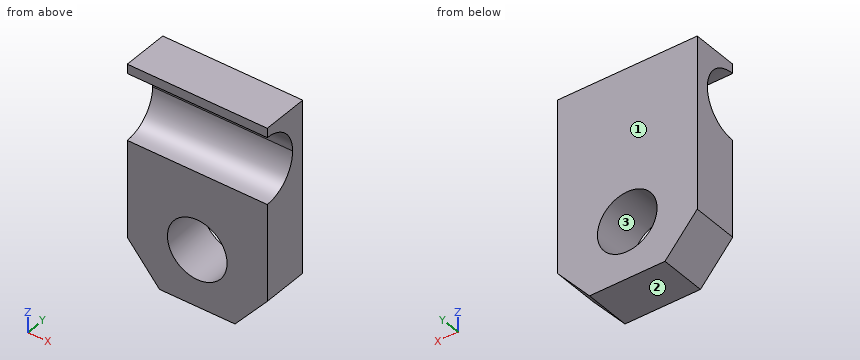
```python
from build123d import *

# Parameters (mm, degrees)
F0_W      = 38.1
F0_H      = 57.15
F1_DEPTH  = 12.7
F3_DEPTH  = 25.4
F7_DEPTH  = 101.6
F9_DEPTH  = 2.54
F10_R     = 8.114992
F11_DEPTH = 25.4


with BuildPart() as f1:
    # F0 (on Front) → F1 (new body)
    with BuildSketch(Plane.XZ):
        Rectangle(F0_W, F0_H)
    extrude(amount=F1_DEPTH)

    # F2 (on face) → F3 (cut)
    with BuildSketch(Plane.XZ.offset(12.7)):
        Polygon((19.05, -18.421547), (10.264741, -28.575), (19.05, -28.575), align=None)
        Polygon((-19.05, -28.575), (-10.264741, -28.575), (-19.05, -18.421547), align=None)
    extrude(amount=-F3_DEPTH, mode=Mode.SUBTRACT)

    # F5 (on face) → F7 (cut)
    with BuildSketch(Plane.YZ.offset(19.05)):
        with BuildLine():
            ThreePointArc((-12.7, 7.877494), (-6.281125, 10.536279), (-3.62234, 16.955154))
            ThreePointArc((-3.62234, 16.955154), (-6.281125, 23.374029), (-12.7, 26.032814))
            Line((-12.7, 26.032814), (-12.7, 7.877494))
        make_face()
        with BuildLine():
            Line((-12.7, 7.877494), (-12.7, 26.032814))
            ThreePointArc((-12.7, 26.032814), (-21.77766, 16.955154), (-12.7, 7.877494))
        make_face()
    extrude(amount=-F7_DEPTH, mode=Mode.SUBTRACT)

    # F8 (on face) → F9 (join)
    with BuildSketch(Plane(origin=(0, 0, 0), x_dir=(-1, 0, 0), z_dir=(0, 1, 0))):
        Polygon((-19.05, 28.575), (-19.05, -18.421547), (-10.264741, -28.575), (10.264741, -28.575), (19.05, -18.421547), (19.05, 28.575), align=None)
    extrude(amount=-F9_DEPTH)

    # F10 (on face) → F11 (cut)
    with BuildSketch(Plane.XZ.offset(12.7)):
        with Locations((0, -13.105877)):
            Circle(F10_R)
    extrude(amount=-F11_DEPTH, mode=Mode.SUBTRACT)


solid = f1.part
```
Work out the finished part from the listing and answer in its coordinate system (mm). Face numbers are marked on the shaded views. Round coordinates to 2 decimals unless told otherwise and drop trailing zeros. Write each loop counter-clockwise with the first axis right and the second up, starting at its lowest first coordinate (ties: lowest second). Pieces come first, ordered by that corner, then holes. Notation, with made-up numbers: (13, 32) -> (47, 32) arc R14 cw to (47, 46) -> close; hole circle Ø11 at (10.5, -14). An arc over 180 degrees is marked (long way). Write each question's results on one line, items separated by ' | '.
Q1. A flat-ended cylindrical pin translates along its axis: P1, Ø12, axis at x = -3.5, z = 17.5, coming from the -Y side. Find the tip coordinate at first contact, or state that the pin passes through.
Data:
P1: y = -6.41
Q2. Section B-B, the plane y = -7.25 is taken. Write down the section's boundary in (x, z) (3 decimals), then the cut area to 3 significant figures.
Data:
outline: (-19.05, -18.422) -> (-10.265, -28.575) -> (10.265, -28.575) -> (19.05, -18.422) -> (19.05, 9.696) -> (-19.05, 9.696) -> close; (-19.05, 24.215) -> (19.05, 24.215) -> (19.05, 28.575) -> (-19.05, 28.575) -> close; hole circle Ø16.23 at (0, -13.106) | area: 1,330 mm^2
Q3. Straight lines are drawn through the part: line 1 along Z through (x, y) = (0, -6.5) (3 decimals); line 2 along Z through (x, y) = (0, -4.75) (3 decimals); line 3 along X through (y, z) = (-8.75, -9). For each, find the intervals that lie inside material, in ascending order. Write a range as [from, to].
Data:
line 1: [-28.575, -21.221], [-4.991, 10.325], [23.586, 28.575] | line 2: [-28.575, -21.221], [-4.991, 12.573], [21.337, 28.575] | line 3: [-19.05, -7], [7, 19.05]
Q4. Section D-D, the plane y = -2.25 is taken. Write down the section's boundary in (x, z) (3 decimals).
Data:
outline: (-19.05, -18.422) -> (-10.265, -28.575) -> (10.265, -28.575) -> (19.05, -18.422) -> (19.05, 28.575) -> (-19.05, 28.575) -> close; hole circle Ø16.23 at (0, -13.106)
Q5. Determine the mould class of the marked faces 1, 2 and 3 for opening direction Z: released by +Z, released by -Z, zero draft, split by the parting line, or undercut.
Data:
face 1: zero draft | face 2: released by -Z | face 3: undercut
